```python
from build123d import *

# Parameters (mm, degrees)
EXTRUDE_1_DEPTH       = 3
SKETCH_2_W            = 7.5
SKETCH_2_H            = 30
SKETCH_3_W            = 7.5
SKETCH_3_H            = 30
SKETCH_4_W            = 7.5
SKETCH_4_H            = 30
SKETCH_5_W            = 7.5
SKETCH_5_H            = 30
SKETCH_6_W            = 7.5
SKETCH_6_H            = 30
SKETCH_7_W            = 7.5
SKETCH_7_H            = 30
SKETCH_8_W            = 7.5
SKETCH_8_H            = 30
SKETCH_9_W            = 7.5
SKETCH_9_H            = 30
SKETCH_10_W           = 7.5
SKETCH_10_H           = 30
SKETCH_11_W           = 7.5
SKETCH_11_H           = 30
HOLE_WIZARD_2_0_2_1_D = 2
FILLET_1_R            = 1
EXTRUDE_START         = 12
SKETCH_14_R           = 7.5
EXTRUDE_2_DEPTH       = 12


with BuildPart() as part:
    # 草图1 → 凸台-拉伸1 (new body)
    with BuildSketch(Plane.XZ.offset(9.693825789)):
        Polygon((-36.617689836, 41.909926554), (-9.984344221, 12.065917083), (69.848381115, 83.310116605), (43.215035499, 113.154126076), align=None)
    extrude(amount=-EXTRUDE_1_DEPTH)

    # 草图2 → 旋转1 (revolve)
    with BuildSketch(Plane(origin=(0, 0, 68.132775199), x_dir=(-1, 0, 0), z_dir=(0, 0, -1)), mode=Mode.PRIVATE) as revolve_1_sk:
        with Locations((-41.57263666, -24.693825789)):
            Rectangle(SKETCH_2_W, SKETCH_2_H)
    revolve(revolve_1_sk.sketch.rotate(Axis((37.82263666, -39.693825789, 68.132775199), (0, 1, 0)), 270), axis=Axis((37.82263666, -39.693825789, 68.132775199), (0, 1, 0)))

    # 草图3 → 旋转2 (revolve)
    with BuildSketch(Plane(origin=(0, 0, 83.054779935), x_dir=(-1, 0, 0), z_dir=(0, 0, -1)), mode=Mode.PRIVATE) as revolve_2_sk:
        with Locations((-28.255963852, -24.693825789)):
            Rectangle(SKETCH_3_W, SKETCH_3_H)
    revolve(revolve_2_sk.sketch.rotate(Axis((24.505963852, -39.693825789, 83.054779935), (0, 1, 0)), 270), axis=Axis((24.505963852, -39.693825789, 83.054779935), (0, 1, 0)))

    # 草图4 → 旋转3 (revolve)
    with BuildSketch(Plane(origin=(0, 0, 97.037286383), x_dir=(-1, 0, 0), z_dir=(0, 0, -1)), mode=Mode.PRIVATE) as revolve_3_sk:
        with Locations((-43.924068825, -24.693825789)):
            Rectangle(SKETCH_4_W, SKETCH_4_H)
    revolve(revolve_3_sk.sketch.rotate(Axis((40.174068825, -39.693825789, 97.037286383), (0, 1, 0)), 270), axis=Axis((40.174068825, -39.693825789, 97.037286383), (0, 1, 0)))

    # 草图5 → 旋转4 (revolve)
    with BuildSketch(Plane(origin=(0, 0, 82.115281647), x_dir=(-1, 0, 0), z_dir=(0, 0, -1)), mode=Mode.PRIVATE) as revolve_4_sk:
        with Locations((-57.240741633, -24.693825789)):
            Rectangle(SKETCH_5_W, SKETCH_5_H)
    revolve(revolve_4_sk.sketch.rotate(Axis((53.490741633, -39.693825789, 82.115281647), (0, 1, 0)), 270), axis=Axis((53.490741633, -39.693825789, 82.115281647), (0, 1, 0)))

    # 草图6 → 旋转5 (revolve)
    with BuildSketch(Plane(origin=(0, 0, 69.072273487), x_dir=(-1, 0, 0), z_dir=(0, 0, -1)), mode=Mode.PRIVATE) as revolve_5_sk:
        with Locations((-12.58785888, -24.693825789)):
            Rectangle(SKETCH_6_W, SKETCH_6_H)
    revolve(revolve_5_sk.sketch.rotate(Axis((8.83785888, -39.693825789, 69.072273487), (0, 1, 0)), 270), axis=Axis((8.83785888, -39.693825789, 69.072273487), (0, 1, 0)))

    # 草图7 → 旋转6 (revolve)
    with BuildSketch(Plane(origin=(0, 0, 55.089767038), x_dir=(-1, 0, 0), z_dir=(0, 0, -1)), mode=Mode.PRIVATE) as revolve_6_sk:
        with Locations((3.080246092, -24.693825789)):
            Rectangle(SKETCH_7_W, SKETCH_7_H)
    revolve(revolve_6_sk.sketch.rotate(Axis((-6.830246092, -39.693825789, 55.089767038), (0, 1, 0)), 270), axis=Axis((-6.830246092, -39.693825789, 55.089767038), (0, 1, 0)))

    # 草图8 → 旋转7 (revolve)
    with BuildSketch(Plane(origin=(0, 0, 41.10726059), x_dir=(-1, 0, 0), z_dir=(0, 0, -1)), mode=Mode.PRIVATE) as revolve_7_sk:
        with Locations((18.748351065, -24.693825789)):
            Rectangle(SKETCH_8_W, SKETCH_8_H)
    revolve(revolve_7_sk.sketch.rotate(Axis((-22.498351065, -39.693825789, 41.10726059), (0, 1, 0)), 270), axis=Axis((-22.498351065, -39.693825789, 41.10726059), (0, 1, 0)))

    # 草图9 → 旋转8 (revolve)
    with BuildSketch(Plane(origin=(0, 0, 54.150268751), x_dir=(-1, 0, 0), z_dir=(0, 0, -1)), mode=Mode.PRIVATE) as revolve_8_sk:
        with Locations((-25.904531688, -24.693825789)):
            Rectangle(SKETCH_9_W, SKETCH_9_H)
    revolve(revolve_8_sk.sketch.rotate(Axis((22.154531688, -39.693825789, 54.150268751), (0, 1, 0)), 270), axis=Axis((22.154531688, -39.693825789, 54.150268751), (0, 1, 0)))

    # 草图10 → 旋转9 (revolve)
    with BuildSketch(Plane(origin=(0, 0, 40.167762303), x_dir=(-1, 0, 0), z_dir=(0, 0, -1)), mode=Mode.PRIVATE) as revolve_9_sk:
        with Locations((-10.236426715, -24.693825789)):
            Rectangle(SKETCH_10_W, SKETCH_10_H)
    revolve(revolve_9_sk.sketch.rotate(Axis((6.486426715, -39.693825789, 40.167762303), (0, 1, 0)), 270), axis=Axis((6.486426715, -39.693825789, 40.167762303), (0, 1, 0)))

    # 草图11 → 旋转10 (revolve)
    with BuildSketch(Plane(origin=(0, 0, 26.185255855), x_dir=(-1, 0, 0), z_dir=(0, 0, -1)), mode=Mode.PRIVATE) as revolve_10_sk:
        with Locations((5.431678257, -24.693825789)):
            Rectangle(SKETCH_11_W, SKETCH_11_H)
    revolve(revolve_10_sk.sketch.rotate(Axis((-9.181678257, -39.693825789, 26.185255855), (0, 1, 0)), 270), axis=Axis((-9.181678257, -39.693825789, 26.185255855), (0, 1, 0)))

    # Ø2.0 (2) 直径孔1 (through all)
    with Locations(Plane(origin=(0, -9.693825789, 0), x_dir=(-1, 0, 0), z_dir=(0, -1, 0))):
        with Locations((-43.014369008, -109.624291383), (9.78367773, -15.595751776), (33.087855144, -41.709260063), (-66.318546422, -83.510783096)):
            Hole(HOLE_WIZARD_2_0_2_1_D / 2)

    # 圆角1
    fillet_1_edges = [part.edges().sort_by_distance(p)[0] for p in [
        (43.215035499, -8.193825789, 113.154126076),
        (69.848381115, -8.193825789, 83.310116605),
        (-9.984344221, -8.193825789, 12.065917083),
        (-36.617689836, -8.193825789, 41.909926554),
    ]]
    fillet(fillet_1_edges, radius=FILLET_1_R)

    # 草图14 → 凸台-拉伸2 (add)
    with BuildSketch(Plane.XZ.offset(39.693825789).offset(EXTRUDE_START)):
        with Locations(Location((40.174068825, 97.037286383, 0), (0, 0, 270))):
            Circle(SKETCH_14_R)
        with Locations(Location((24.505963852, 83.054779935, 0), (0, 0, 270))):
            Circle(SKETCH_14_R)
        with Locations(Location((8.83785888, 69.072273487, 0), (0, 0, 270))):
            Circle(SKETCH_14_R)
        with Locations(Location((-6.830246092, 55.089767038, 0), (0, 0, 270))):
            Circle(SKETCH_14_R)
        with Locations(Location((-22.498351065, 41.10726059, 0), (0, 0, 270))):
            Circle(SKETCH_14_R)
        with Locations(Location((-9.181678257, 26.185255855, 0), (0, 0, 270))):
            Circle(SKETCH_14_R)
        with Locations(Location((6.486426715, 40.167762303, 0), (0, 0, 270))):
            Circle(SKETCH_14_R)
        with Locations(Location((22.154531688, 54.150268751, 0), (0, 0, 270))):
            Circle(SKETCH_14_R)
        with Locations(Location((37.82263666, 68.132775199, 0), (0, 0, 270))):
            Circle(SKETCH_14_R)
        with Locations(Location((53.490741633, 82.115281647, 0), (0, 0, 270))):
            Circle(SKETCH_14_R)
    extrude(amount=-EXTRUDE_2_DEPTH)


solid = part.part
```
Read the model definition and answer for the solid it produces. Units are mm, in the model's axes. A direction names the side the tool comes from. Coordinates: 2 decimals unless noted, no trailing zeros. Loops run counter-clockwise (first coordinate to the right, second up) from the corner with the lowest first, then second, coordinate; pieces in that order, holes last. Notation, with made-up numbers: (43, 28.5) -> (100, 28.5) arc R24 ccw to (100, 61.5) -> close; hole circle Ø9 at (76, 37). An arc over 180 degrees is marked (long way). Return JSON: item names as keys, results as strings.
Item 1: Find the intervals of material crossed by probe 1 along Y at (x, z) = (12, 56); probe 2 along X at (y, z) = (-26.5, 96.5); probe 3 along X at (y, z) = (-29.5, 54), in increasing order.
Answers:
{"probe 1": "y = -9.69 to -6.69", "probe 2": "x = 32.69 to 47.65", "probe 3": "x = -14.25 to 0.59, 14.66 to 29.65"}
Item 2: Find section B-B (z = 97.5). Determine the outline of the cut face in (x, y), plus the area to 3 significant figures.
Answers:
{"outline": "(25.67, -9.69) -> (32.69, -9.69) -> (32.69, -51.69) -> (47.66, -51.69) -> (47.66, -9.69) -> (57.19, -9.69) -> (57.19, -6.69) -> (25.67, -6.69) -> close", "area": "723 mm2"}
Item 3: Find section A-A (y = -42.5). Count the separate pieces of the cut face and the enclosed holes in it, plus the area to 3 significant figures.
Answers:
{"separate pieces": "10", "enclosed holes": "0", "area": "1,770 mm2"}
Item 4: Flat-ended cylindrical pins translate along their axes: P1, Ø5, axis at x = -24, y = -28.5, coming from the -Z side; P2, Ø1.2, axis at x = -33.09, z = 41.71, coming from the -Y side; P3, Ø6, axis at y = -42.5, z = 99.5, coming from the +X side; P4, Ø1, axis at y = -20.5, z = 37, coming from the -X side. Find the tip coordinate at first contact, or state that the pin passes through.
Answers:
{"P1": "stops at z = 33.61", "P2": "passes through", "P3": "stops at x = 47.67", "P4": "stops at x = -29.07"}
Item 5: For a pull along X with two mould halves and no side action, classify faces 3 (the cylindrical face through (-15.015, -30.4, 41.602)), 4 (the flat face through (-7, -51.694, 55)), 5 (the flat face through (3.847, -8.215, 78.021)) as +X half, -X half, draft (parallel to the pull), parting line (faces both ways), or undercut.
Answers:
{"face 3": "undercut", "face 4": "draft", "face 5": "-X half"}
Item 6: Find section C-C (x = 50). Determine the outline of the cut face in (y, z).
Answers:
{"outline": "(-51.69, 75.48) -> (-9.69, 75.48) -> (-9.69, 65.6) -> (-6.69, 65.6) -> (-6.69, 105.55) -> (-9.69, 105.55) -> (-9.69, 88.75) -> (-51.69, 88.75) -> close"}
Item 7: For faces 1 (the flat face through (-22, -51.694, 41)), 2 (the cylindrical face through (29.64, -30.4, 54.64)), determine the directions among +Z, -Z, +X, -X, +Y, -Y from which every point of the face is accessible in a straight line to the end or side of a thin tool.
Answers:
{"face 1": "+Z, -Z, +X, -X, -Y", "face 2": "-Y"}
Item 8: Find section D-D (z = 55.5). Determine the outline of the cut face in (x, y).
Answers:
{"outline": "(-21.39, -9.69) -> (-14.32, -9.69) -> (-14.32, -51.69) -> (0.66, -51.69) -> (0.66, -9.69) -> (14.78, -9.69) -> (14.78, -51.69) -> (29.53, -51.69) -> (29.53, -9.69) -> (38.69, -9.69) -> (38.69, -6.69) -> (-21.39, -6.69) -> close"}
